from build123d import *

# Parameters (mm, degrees)
PAD_DEPTH          = 7
SKETCH001_R        = 3.3
PAD001_DEPTH       = 11
SKETCH002_R        = 4.2
PAD002_DEPTH       = 2
SKETCH003_W        = 0.5
SKETCH003_H        = 4.2
PAD003_DEPTH       = 1
POLARPATTERN_COUNT = 12


with BuildPart() as part:
    # Sketch (on XY_Plane of Origin) → Pad (new body)
    with BuildSketch(Plane.XY):
        Polygon((6.581793, 0), (3.290897, 5.7), (-3.290897, 5.7), (-6.581793, 0), (-3.290897, -5.7), (3.290897, -5.7), align=None)
    extrude(amount=PAD_DEPTH)

    # Sketch001 (on Face8 of Pad) → Pad001 (join)
    with BuildSketch(Plane.XY.offset(7)):
        Circle(SKETCH001_R)
    extrude(amount=PAD001_DEPTH)

    # Sketch002 (on Face10 of Pad001) → Pad002 (join)
    with BuildSketch(Plane.XY.offset(18)):
        Circle(SKETCH002_R)
    extrude(amount=PAD002_DEPTH)

    # Sketch003 (on Face12 of Pad002) → Pad003 (join)
    with BuildSketch(Plane.XY.offset(20)):
        with Locations((0, 2.1)):
            Rectangle(SKETCH003_W, SKETCH003_H)
    pad003 = extrude(amount=PAD003_DEPTH)

    # PolarPattern: Pad003 ×12 about axis
    polarpattern_axis = Axis((0, 0, 20), (0, 0, 1))
    for i in range(1, POLARPATTERN_COUNT):
        add(pad003.rotate(polarpattern_axis, i * 360 / POLARPATTERN_COUNT))

    # Sketch004 (on YZ_Plane of Origin) → Groove (revolve, cut)
    with BuildSketch(Plane.YZ):
        Polygon((0, 21), (4.440189, 20.5), (4.440189, 21), align=None)
    revolve(axis=Axis((0, 0, 0), (0, 0, 1)), mode=Mode.SUBTRACT)


solid = part.part
Check sheet for the modelled part. Datum: model origin and axes. Units: mm. A direction names the side the tool comes from. Coordinates: 2 decimals unless noted, no trailing zeros. Loops run counter-clockwise (first coordinate to the right, second up) from the corner with the lowest first, then second, coordinate; pieces in that order, holes last. Notation, with made-up numbers: (40.25, 40.25) -> (77.25, 40.25) arc R15 cw to (77.25, 66.25) -> close; hole circle Ø10 at (12.5, 18.25). An arc over 180 degrees is marked (long way). Write item = value, one per line. Start each with the question number.
1. Section check C-C on y = 5. Record the cut outline in (x, z), then the cut area to 3 significant figures.
2. Tool access check on faces 5 (the flat face through (-1, -3, 20)), 6 (the flat face through (-4.913, 2.89, 3.451)), 7 (the flat face through (-3, -1, 20)), 8 (the flat face through (-2, 2, 20)). Record the directions out of +Z, -Z, +X, -X, +Y, -Y that give a thin tool (end or side, any length) a straight path to the whole face; none if there is none.
3. Depth check by flat-ended pin: P1, Ø3, axis at x = 1.5, y = 2, coming from the +Z side; P2, Ø2, axis at x = -2.5, y = -2.5, coming from the +Z side; P3, Ø0.6, axis at x = 0, z = 20.5, coming from the +Y side. Enter the tip coordinate at first touch or a pass-through.
4. Draft check along Y on faces 1 (the flat face through (1.5, 2.1, 20.3)), 2 (the cylindrical face through (-2.43, 2.23, 12.42)), 3 (the flat face through (-2.5, -0.25, 20.3)), 4 (the flat face through (4.96, 2.81, 3.45)). Enter one of: released by +Y, released by -Y, zero draft, split by the parting line, or undercut.
5. Material ranges on line 1 (Z direction, x = -2.75, y = -4.75); line 2 (Z direction, x = 1.5, y = 1.5); line 3 (X direction, y = 3.25, z = 2.5), recorded low to high.
6. Section check A-A on z = 3.25. Record the cut outline in (x, y), then the cut area to 3 significant figures.
7. Section check B-B on x = -4.5. Record the cut outline in (y, z).
8. Section check D-D on z = 19.75. Record the cut outline in (x, y), then the cut area to 3 significant figures.
Responses:
q1.outline = (-3.7, 0) -> (3.7, 0) -> (3.7, 7) -> (-3.7, 7) -> close
q1.area = 51.7 mm2
q2.face_5 = +Z, -Y
q2.face_6 = +Z, -Z, -X, +Y
q2.face_7 = +Z, -X
q2.face_8 = +Z
q3.P1 = 20.89
q3.P2 = 20.7
q3.P3 = 4.2
q4.face_1 = undercut
q4.face_2 = split by the parting line
q4.face_3 = undercut
q4.face_4 = released by +Y
q5.line_1 = 0 to 7
q5.line_2 = 0 to 20
q5.line_3 = -4.71 to 4.71
q6.outline = (-6.58, 0) -> (-3.29, -5.7) -> (3.29, -5.7) -> (6.58, 0) -> (3.29, 5.7) -> (-3.29, 5.7) -> close
q6.area = 113 mm2
q7.outline = (-3.61, 0) -> (3.61, 0) -> (3.61, 7) -> (-3.61, 7) -> close
q8.outline = circle Ø8.4 at (0, 0)
q8.area = 55.4 mm2
